Read the model definition and answer for the solid it produces. Units are mm, in the model's axes. A direction names the side the tool comes from. Round coordinates to 2 decimals unless told otherwise and drop trailing zeros. Order: outer loops, then holes, each group sorted by start corner. A loop starts at its lowest first (then second) coordinate and runs counter-clockwise, first axis right, second up.
from build123d import *

# Parameters (mm, degrees)
F0_W     = 4.5
F0_H     = 2
F0_H_2   = 4.5
F0_W_2   = 20
F1_DEPTH = 7.36
F2_R     = 2.6
F3_DEPTH = 50
F4_SIZE2 = 4.0192378865
F4_SIZE  = 15
F5_R     = 5
F6_SIZE  = 2


with BuildPart() as f1:
    # F0 (on Front) → F1 (new body, symmetric)
    with BuildSketch(Plane.XZ):
        with Locations((2.25, 1)):
            Rectangle(F0_W, F0_H)
        with Locations((2.25, -2.25)):
            Rectangle(F0_W, F0_H_2)
        with Locations((14.5, -2.25)):
            Rectangle(F0_W_2, F0_H_2)
        Polygon((-15.7, 2), (0, 2), (4.5, 2), (4.5, 6.5), (-15.7, 6.5), align=None)
    extrude(amount=F1_DEPTH, both=True)

    # F2 (on face) → F3 (cut, symmetric)
    with BuildSketch(Plane.XY):
        with Locations((14.5, 0)):
            Circle(F2_R)
    extrude(amount=F3_DEPTH, both=True, mode=Mode.SUBTRACT)

    # F4
    f4_edges = [f1.edges().sort_by_distance(p)[0] for p in [
        (0, 0, 2),
    ]]
    f4_side = f1.faces().sort_by_distance((-7.85, 0, 2))[0]
    chamfer(f4_edges, length=F4_SIZE, length2=F4_SIZE2, reference=f4_side)

    # F5
    f5_edges = [f1.edges().sort_by_distance(p)[0] for p in [
        (-15.7, 7.36, 4.25),
        (-15.7, -7.36, 4.25),
        (24.5, 7.36, -2.25),
        (24.5, -7.36, -2.25),
    ]]
    fillet(f5_edges, radius=F5_R)

    # F6
    f6_edges = [f1.edges().sort_by_distance(p)[0] for p in [
        (4.5, 0, 0),
    ]]
    chamfer(f6_edges, length=F6_SIZE)


solid = f1.part
Q1. Straight lines are drawn through the part: probe 1 along Y at (x, z) = (14.5, -2.3); probe 2 along Z at (x, y) = (21.5, 4.5); probe 3 along Y at (x, z) = (13, -2.75). For each, find the intervals that lie inside material, in ascending order.
Outcome:
probe 1: y = -7.36 to -2.6, 2.6 to 7.36
probe 2: z = -4.5 to 0
probe 3: y = -7.36 to -2.12, 2.12 to 7.36
Q2. For a pull along Y with two mould halves and no side action, classify faces 4 (the face through (16.98, 0.78, -2.22)), 5 (the face through (4, -7.36, 1)), 6 (the face through (24.5, 0, -2)) as released by +Y, released by -Y, zero draft, split by the parting line, or undercut.
Outcome:
face 4: undercut
face 5: released by -Y
face 6: zero draft
Q3. A cutting plane is placed at C-C, the plane z = -3.5. Give the vertices of the cut face in (x, y).
Outcome:
outline: (0, -7.36) - (19.5, -7.36) arc R5 ccw to (24.5, -2.36) - (24.5, 2.36) arc R5 ccw to (19.5, 7.36) - (0, 7.36) - close; hole circle Ø5.2 at (14.5, 0)
Q4. For faces 1 (the face through (4, 7.36, 1)), 2 (the face through (0, 0, -3)), 3 (the face through (17.4, -0.1, 0)), determine the directions among +Z, -Z, +X, -X, +Y, -Y from which every point of the face is accessible in a straight line to the end or side of a thin tool.
Outcome:
face 1: +Z, -Z, +X, -X, +Y
face 2: -Z, -X, +Y, -Y
face 3: +Z, +X, +Y, -Y
Q5. A cutting plane is placed at B-B, the plane y = 0. Give the vertices of the cut face in (x, z).
Outcome:
outline: (-15.7, 2) - (-15, 2) - (0, -2.02) - (0, -4.5) - (11.9, -4.5) - (11.9, 0) - (6.5, 0) - (4.5, 2) - (4.5, 6.5) - (-15.7, 6.5) - close; (17.1, -4.5) - (24.5, -4.5) - (24.5, 0) - (17.1, 0) - close
Q6. Flat-ended cylindrical pins translate along their axes: pin 1 (2 mm diameter, centred on y = 3.5, z = 4.5, fed in from +X); pin 2 (5 mm diameter, centred on x = -8.5, y = -5.5, fed in from -Z); pin 3 (4 mm diameter, centred on x = 19.5, z = 3, fed in from -Y); pin 4 (4.5 mm diameter, centred on x = 19, y = 2, fed in from +Z). Find the tip coordinate at first contact, or state that the pin passes through.
Outcome:
pin 1: stops at x = 4.5
pin 2: stops at z = -0.41
pin 3: passes through
pin 4: stops at z = 0
Q7. A cutting plane is placed at D-D, the plane z = 3. Give the vertices of the cut face in (x, y).
Outcome:
outline: (-15.7, -2.36) arc R5 ccw to (-10.7, -7.36) - (4.5, -7.36) - (4.5, 7.36) - (-10.7, 7.36) arc R5 ccw to (-15.7, 2.36) - close
Q8. A cutting plane is placed at A-A, the plane x = 14.5. Give the vertices of the cut face in (y, z).
Outcome:
outline: (-7.36, -4.5) - (-2.6, -4.5) - (-2.6, 0) - (-7.36, 0) - close; (2.6, -4.5) - (7.36, -4.5) - (7.36, 0) - (2.6, 0) - close
